```python
from build123d import *

# Parameters (mm, degrees)
SKETCH1_W           = 180
SKETCH1_H           = 20
SKETCH1_R           = 5
BOSS_EXTRUDE1_DEPTH = 5
BOSS_EXTRUDE4_START = -10
SKETCH2_R           = 2
BOSS_EXTRUDE4_DEPTH = 5
SKETCH2_3_R         = 2
BOSS_EXTRUDE5_DEPTH = 5
BOSS_EXTRUDE6_START = 10
SKETCH2_4_R         = 2
BOSS_EXTRUDE6_DEPTH = 5
SKETCH2_5_R         = 2
BOSS_EXTRUDE7_DEPTH = 5
SKETCH1_3_R         = 5
BOSS_EXTRUDE8_DEPTH = 10
SKETCH3_W           = 6
SKETCH3_H           = 4
BOSS_EXTRUDE9_DEPTH = 3


with BuildPart() as part:
    # Sketch1 → Boss-Extrude1 (new body)
    # profile 1 of 2: a face of its own
    with BuildSketch(Plane(origin=(0, 0, 0), x_dir=(1, 0, 0), z_dir=(0, 1, 0))):
        Rectangle(SKETCH1_W, SKETCH1_H)
        Circle(SKETCH1_R, mode=Mode.SUBTRACT)
    # profile 2 of 2: a face of its own
    with BuildSketch(Plane(origin=(0, 0, 0), x_dir=(1, 0, 0), z_dir=(0, 1, 0))):
        Circle(SKETCH1_R)
    extrude(amount=BOSS_EXTRUDE1_DEPTH)

    # Sketch2 → Boss-Extrude4 (add)
    # profile 1 of 2: a face of its own
    with BuildSketch(Plane.XY.offset(BOSS_EXTRUDE4_START)):
        with BuildLine():
            ThreePointArc((-90, 13), (-85, 18), (-80, 13))
            Line((-80, 13), (-80, 5))
            Line((-80, 5), (-90, 5))
            Line((-90, 5), (-90, 13))
        make_face()
        with Locations((-85, 13)):
            Circle(SKETCH2_R, mode=Mode.SUBTRACT)
    # profile 2 of 2: a face of its own
    with BuildSketch(Plane.XY.offset(BOSS_EXTRUDE4_START)):
        with Locations((-85, 13)):
            Circle(SKETCH2_R)
    extrude(amount=BOSS_EXTRUDE4_DEPTH)

    # Sketch2<3> → Boss-Extrude5 (add)
    with BuildSketch(Plane.XY):
        with Locations((-85, 13)):
            Circle(SKETCH2_3_R)
    extrude(amount=-BOSS_EXTRUDE5_DEPTH)

    # Sketch2<4> → Boss-Extrude6 (add)
    # profile 1 of 2: a face of its own
    with BuildSketch(Plane.XY.offset(BOSS_EXTRUDE6_START)):
        with BuildLine():
            Line((90, 5), (90, 13))
            ThreePointArc((90, 13), (85, 18), (80, 13))
            Line((80, 13), (80, 5))
            Line((80, 5), (90, 5))
        make_face()
        with Locations((85, 13)):
            Circle(SKETCH2_4_R, mode=Mode.SUBTRACT)
    # profile 2 of 2: a face of its own
    with BuildSketch(Plane.XY.offset(BOSS_EXTRUDE6_START)):
        with Locations((85, 13)):
            Circle(SKETCH2_4_R)
    extrude(amount=-BOSS_EXTRUDE6_DEPTH)

    # Sketch2<5> → Boss-Extrude7 (add)
    with BuildSketch(Plane.XY):
        with Locations((85, 13)):
            Circle(SKETCH2_5_R)
    extrude(amount=BOSS_EXTRUDE7_DEPTH)

    # Sketch1<3> → Boss-Extrude8 (add)
    with BuildSketch(Plane(origin=(0, 0, 0), x_dir=(1, 0, 0), z_dir=(0, 1, 0))):
        with Locations(Location((0, 0, 0), (0, 0, 270))):
            Circle(SKETCH1_3_R)
    extrude(amount=-BOSS_EXTRUDE8_DEPTH)

    # Sketch3 → Boss-Extrude9 (add)
    with BuildSketch(Plane.XY.offset(10)):
        with Locations((22, -2)):
            Rectangle(SKETCH3_W, SKETCH3_H)
    extrude(amount=-BOSS_EXTRUDE9_DEPTH)


solid = part.part
```
Work out the finished part from the listing and answer in its coordinate system (mm). A direction names the side the tool comes from. Round coordinates to 2 decimals unless told otherwise and drop trailing zeros. Order: outer loops, then holes, each group sorted by start corner. A loop starts at its lowest first (then second) coordinate and runs counter-clockwise, first axis right, second up.
Q1. A cutting plane is placed at B-B, the plane x = 0. Determine the outline of the cut face in (y, z), then the cut area to 3 significant figures.
Solution:
outline: (-10, -5) - (0, -5) - (0, -10) - (5, -10) - (5, 10) - (0, 10) - (0, 5) - (-10, 5) - close
area: 200 mm2
Q2. A tool of negligible diameter and unlimited length cuts with its end or side. For faces 4 (the cylindrical face through (-4.88, -4.93, -1.08)), 5 (the flat face through (-80, 9, -8)), 6 (the flat face through (-85, 10, -5)), 7 (the flat face through (-85, 13, 0)), 8 (the flat face through (80, 9, 8)), from which of +Z, -Z, +X, -X, +Y, -Y can it reach the whole face along a straight path? Write none if from no direction.
Solution:
face 4: -Y
face 5: +Z, -Z, +X, +Y
face 6: +Z
face 7: +Z, -X, +Y
face 8: +Z, -Z, -X, +Y
Q3. A cutting plane is placed at A-A, the plane y = 7.75. Determine the outline of the cut face in (x, z).
Solution:
outline: (-90, -10) - (-80, -10) - (-80, -5) - (-90, -5) - close; (80, 5) - (90, 5) - (90, 10) - (80, 10) - close
Q4. A cutting plane is placed at C-C, the plane z = -3.5. Determine the outline of the cut face in (x, y), then the cut area to 3 significant figures.
Solution:
outline: (-90, 0) - (-3.57, 0) - (-3.57, -10) - (3.57, -10) - (3.57, 0) - (90, 0) - (90, 5) - (-90, 5) - close; circle Ø4 at (-85, 13)
area: 984 mm2
Q5. The mould has two halves that part along Y. Classify faces 1 (the cylindrical face through (86.908, 13.601, 2.465)), 2 (the cylindrical face through (-85, 18, -8)), 3 (the flat face through (25, -2, 9)): pulls with the +Y half, pulls with the -Y half, needs draft (parallel to the pull), parting line crosses it, or undercut.
Solution:
face 1: undercut
face 2: pulls with the +Y half
face 3: needs draft
Q6. Find the intervals of material crossed by line 1 along Y through (x, z) = (-42.5, -0.25); line 2 along X through (y, z) = (11.5, 7.25); line 3 along X through (y, z) = (12, 3.75), in increasing order.
Solution:
line 1: y = 0 to 5
line 2: x = 80 to 90
line 3: x = 83.27 to 86.73
Q7. Given pin 1 Ø2.5 at (y, z) = (9, 7.5) entering from -X; pin 2 Ø0.9 at (y, z) = (-1, 8) entering from +X; pin 3 Ø2 at (x, y) = (84.5, 13) entering from -Z, each flat-ended and moving along its own axis, determine where each tip first touches the part or whether it passes through.
Solution:
pin 1: stops at x = 80
pin 2: stops at x = 25
pin 3: stops at z = 0
Q8. A cutting plane is placed at D-D, the plane x = 85. Determine the outline of the cut face in (y, z), then the cut area to 3 significant figures.
Solution:
outline: (0, -10) - (5, -10) - (5, 5) - (11, 5) - (11, 0) - (15, 0) - (15, 5) - (18, 5) - (18, 10) - (0, 10) - close
area: 185 mm2
